Could you check a few things on this model? Use its own coordinates, in mm. Face numbers are marked on the shaded views. A direction names the side the tool comes from. Give positions to 0.01 mm unless a question says otherwise; leave off trailing zeros. Write each loop counter-clockwise with the first axis right and the second up, starting at its lowest first coordinate (ties: lowest second). Pieces come first, ordered by that corner, then holes. Notation, with made-up numbers: (44, 45.5) - (80, 45.5) arc R32 cw to (80, 79.5) - close; hole circle Ø3 at (22, -23.5). An arc over 180 degrees is marked (long way). Answer in a Markdown table with one row per item.
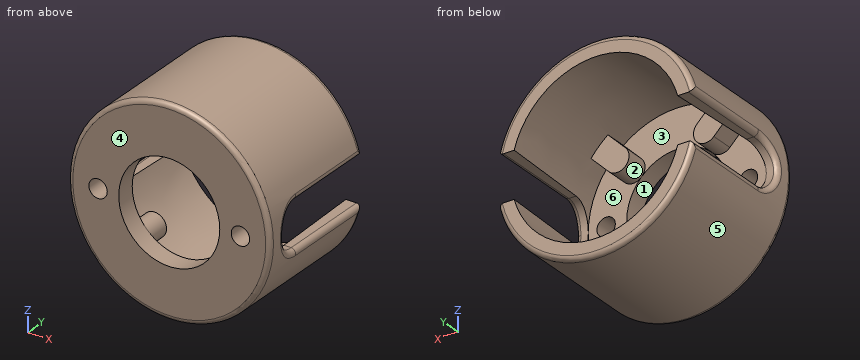
from build123d import *

# Parameters (mm, degrees)
SKETCH1_R           = 11
BOSS_EXTRUDE1_DEPTH = 14.8
SKETCH2_R           = 9.25
CUT_EXTRUDE1_DEPTH  = 12.7
CUT_EXTRUDE1_TAPER  = -2
CUT_EXTRUDE2_REACH  = 4.1
SKETCH3_R           = 5.5
BOSS_EXTRUDE2_DEPTH = 2.5
CUT_EXTRUDE3_DEPTH  = 23
CUT_EXTRUDE4_REACH  = 16.8
SKETCH7_R           = 1
FILLET1_R           = 0.5


with BuildPart() as part:
    # Sketch1 → Boss-Extrude1 (new body)
    with BuildSketch(Plane(origin=(0, 0, 0), x_dir=(1, 0, 0), z_dir=(0, 1, 0))):
        Circle(SKETCH1_R)
    extrude(amount=BOSS_EXTRUDE1_DEPTH)

    # Sketch2 → Cut-Extrude1 (cut)
    with BuildSketch(Plane(origin=(0, 14.8, 0), x_dir=(1, 0, 0), z_dir=(0, 1, 0))):
        Circle(SKETCH2_R)
    extrude(amount=-CUT_EXTRUDE1_DEPTH, taper=CUT_EXTRUDE1_TAPER, mode=Mode.SUBTRACT)

    # Sketch3 → Cut-Extrude2 (cut, up to next)
    with BuildSketch(Plane(origin=(0, 2.1, 0), x_dir=(1, 0, 0), z_dir=(0, 1, 0)), mode=Mode.PRIVATE) as cut_extrude2_sk1:
        Circle(SKETCH3_R)
    cut_extrude2_tool1 = extrude(cut_extrude2_sk1.sketch, amount=-CUT_EXTRUDE2_REACH, mode=Mode.PRIVATE) & part.part
    add(cut_extrude2_tool1.solids().sort_by_distance((0, 2.1, 0))[0], mode=Mode.SUBTRACT)

    # Sketch4 → Boss-Extrude2 (add)
    with BuildSketch(Plane(origin=(0, 2.1, 0), x_dir=(1, 0, 0), z_dir=(0, 1, 0))):
        with BuildLine():
            Line((3.889087297, 5.727564928), (5.873176864, 7.711654495))
            ThreePointArc((5.873176864, 7.711654495), (6.85433518, 6.85433518), (7.711654495, 5.873176864))
            Line((7.711654495, 5.873176864), (5.727564928, 3.889087297))
            ThreePointArc((5.727564928, 3.889087297), (3.889087297, 3.889087297), (3.889087297, 5.727564928))
        make_face()
        with BuildLine():
            Line((3.889087297, -5.727564928), (5.873176864, -7.711654495))
            ThreePointArc((5.873176864, -7.711654495), (6.85433518, -6.85433518), (7.711654495, -5.873176864))
            Line((7.711654495, -5.873176864), (5.727564928, -3.889087297))
            ThreePointArc((5.727564928, -3.889087297), (3.889087297, -3.889087297), (3.889087297, -5.727564928))
        make_face()
        with BuildLine():
            Line((-5.727564928, -3.889087297), (-7.711654495, -5.873176864))
            ThreePointArc((-7.711654495, -5.873176864), (-6.85433518, -6.85433518), (-5.873176864, -7.711654495))
            Line((-5.873176864, -7.711654495), (-3.889087297, -5.727564928))
            ThreePointArc((-3.889087297, -5.727564928), (-3.889087297, -3.889087297), (-5.727564928, -3.889087297))
        make_face()
        with BuildLine():
            Line((-3.889087297, 5.727564928), (-5.873176864, 7.711654495))
            ThreePointArc((-5.873176864, 7.711654495), (-6.85433518, 6.85433518), (-7.711654495, 5.873176864))
            Line((-7.711654495, 5.873176864), (-5.727564928, 3.889087297))
            ThreePointArc((-5.727564928, 3.889087297), (-3.889087297, 3.889087297), (-3.889087297, 5.727564928))
        make_face()
    extrude(amount=BOSS_EXTRUDE2_DEPTH)

    # Sketch6 → Cut-Extrude3 (cut, through all)
    with BuildSketch(Plane.ZY.offset(11)):
        with BuildLine():
            Line((-2.5, 4.6), (-2.5, 14.8))
            Line((-2.5, 14.8), (2.5, 14.8))
            Line((2.5, 14.8), (2.5, 4.6))
            ThreePointArc((2.5, 4.6), (0, 2.1), (-2.5, 4.6))
        make_face()
    extrude(amount=-CUT_EXTRUDE3_DEPTH, mode=Mode.SUBTRACT)

    # Sketch7 → Cut-Extrude4 (cut, up to next)
    with BuildSketch(Plane.XZ, mode=Mode.PRIVATE) as cut_extrude4_sk1:
        with Locations((7.75, 0)):
            Circle(SKETCH7_R)
    cut_extrude4_tool1 = extrude(cut_extrude4_sk1.sketch, amount=-CUT_EXTRUDE4_REACH, mode=Mode.PRIVATE) & part.part
    add(cut_extrude4_tool1.solids().sort_by_distance((7.75, 0, 0))[0], mode=Mode.SUBTRACT)
    # Sketch7 → Cut-Extrude4 (cut, up to next)
    with BuildSketch(Plane.XZ, mode=Mode.PRIVATE) as cut_extrude4_sk2:
        with Locations((-7.75, 0)):
            Circle(SKETCH7_R)
    cut_extrude4_tool2 = extrude(cut_extrude4_sk2.sketch, amount=-CUT_EXTRUDE4_REACH, mode=Mode.PRIVATE) & part.part
    add(cut_extrude4_tool2.solids().sort_by_distance((-7.75, 0, 0))[0], mode=Mode.SUBTRACT)

    # Fillet1
    fillet1_edges = [part.edges().sort_by_distance(p)[0] for p in [
        (-11, 0, 0),
        (0, 14.8, -11),
        (0, 14.8, 11),
        (-10.712142643, 9.7, -2.5),
        (10.712142643, 9.7, -2.5),
        (-10.712142643, 9.7, 2.5),
        (10.712142643, 9.7, 2.5),
        (10.857017021, 2.832284274, 1.767818206),
        (-11, 2.1, 0),
    ]]
    fillet(fillet1_edges, radius=FILLET1_R)


solid = part.part
1) We'd pull the mould along X, two halves only. Please class the marked faces 4, 5 and 6: +X half, -X half, draft (parallel to the pull), parting line (faces both ways), or undercut.
Check values:
| item | result |
|---|---|
| face 4 | draft |
| face 5 | parting line |
| face 6 | undercut |
2) If I drill on line 1 (Z direction, x = 0, y = 1.3); line 2 (Y direction, x = 6, z = 4.5); line 3 (X direction, y = 3.5, z = 6.75), over which ranges is the centre line in solid material (lowest first)?
Check values:
| item | result |
|---|---|
| line 1 | z = -11 to -5.5, 5.5 to 11 |
| line 2 | y = 0 to 4.6 |
| line 3 | x = -8.69 to -4.91, 4.91 to 8.69 |
3) Imagine slicing it at C-C (y = 10). List the corners of the cut face in (x, z) for me.
Check values:
| item | result |
|---|---|
| outline | (-10.54, -3.14) arc R11 ccw to (10.54, -3.14) arc R0.5 ccw to (10.06, -2.5) - (9.08, -2.5) arc R9.42 cw to (-9.08, -2.5) - (-10.06, -2.5) arc R0.5 ccw to start; (-10.54, 3.14) arc R0.5 ccw to (-10.06, 2.5) - (-9.08, 2.5) arc R9.42 cw to (9.08, 2.5) - (10.06, 2.5) arc R0.5 ccw to (10.54, 3.14) arc R11 ccw to start |
4) On a 3-axis mill with a long thin cutter (end or side, diameter ignored), from which of +Z, -Z, +X, -X, +Y, -Y can I reach the whole of each face in a straight line? I mean the marked faces 1, 2 and 3. Say none if no direction works.
Check values:
| item | result |
|---|---|
| face 1 | +Y, -Y |
| face 2 | +Y |
| face 3 | none |
5) Imagine slicing it at A-A (x = 0). List the corners of the cut face in (y, z) for me.
Check values:
| item | result |
|---|---|
| outline | (0, -10.5) arc R0.5 ccw to (0.5, -11) - (14.3, -11) arc R0.5 ccw to (14.8, -10.5) - (14.8, -9.25) - (2.1, -9.69) - (2.1, -5.5) - (0, -5.5) - close; (0, 5.5) - (2.1, 5.5) - (2.1, 9.69) - (14.8, 9.25) - (14.8, 10.5) arc R0.5 ccw to (14.3, 11) - (0.5, 11) arc R0.5 ccw to (0, 10.5) - close |
6) Imagine slicing it at B-B (y = 13). List the corners of the cut face in (x, z) for me.
Check values:
| item | result |
|---|---|
| outline | (-10.54, -3.14) arc R11 ccw to (10.54, -3.14) arc R0.5 ccw to (10.06, -2.5) - (8.97, -2.5) arc R9.31 cw to (-8.97, -2.5) - (-10.06, -2.5) arc R0.5 ccw to start; (-10.54, 3.14) arc R0.5 ccw to (-10.06, 2.5) - (-8.97, 2.5) arc R9.31 cw to (8.97, 2.5) - (10.06, 2.5) arc R0.5 ccw to (10.54, 3.14) arc R11 ccw to start |
7) Will these pins go through, and if not, where does the flat tip stop? P1, Ø0.6, axis at x = 9.5, y = 12, coming from the +Z side; P2, Ø2, axis at y = 2.5, z = 8, coming from the -X side; P3, Ø3, axis at x = 1.5, z = 6.5, coming from the +Y side.
Check values:
| item | result |
|---|---|
| P1 | stops at z = 6.03 |
| P2 | stops at x = -8.49 |
| P3 | stops at y = 2.1 |
